Model file for the job. Use its own axes, mm. A direction names the side the tool comes from. Give positions to 0.01 mm unless a question says otherwise; leave off trailing zeros. Loops run counter-clockwise (first coordinate to the right, second up) from the corner with the lowest first, then second, coordinate; pieces in that order, holes last. Notation, with made-up numbers: (10, 72.25) - (43, 72.25) arc R16 ccw to (43, 77.25) - close; hole circle Ø3 at (-3.5, -10). An arc over 180 degrees is marked (long way). Use a Markdown table: item, result.
from build123d import *

# Parameters (mm, degrees)
F0_R     = 40
F0_R_2   = 11
F1_DEPTH = 9
F2_R     = 1
F3_SIZE  = 1
F9_DEPTH = 2.5


with BuildPart() as f1:
    # F0 (on Top) → F1 (new body)
    with BuildSketch(Plane.XY):
        Circle(F0_R)
        Circle(F0_R_2, mode=Mode.SUBTRACT)
    extrude(amount=F1_DEPTH)

    # F2
    f2_edges = [f1.edges().sort_by_distance(p)[0] for p in [
        (-11, 0, 9),
    ]]
    fillet(f2_edges, radius=F2_R)

    # F3
    f3_edges = [f1.edges().sort_by_distance(p)[0] for p in [
        (-11, 0, 0),
    ]]
    chamfer(f3_edges, length=F3_SIZE)

    # F8 (on face) → F9 (join, symmetric)
    with BuildSketch(Plane.XY.offset(4.5)):
        with BuildLine():
            Line((-12, 1.5), (-12, -1.5))
            Line((-12, -1.5), (-10, -1.5))
            ThreePointArc((-10, -1.5), (-9.292893, -1.207107), (-9, -0.5))
            Line((-9, -0.5), (-9, 0.5))
            ThreePointArc((-9, 0.5), (-9.292893, 1.207107), (-10, 1.5))
            Line((-10, 1.5), (-12, 1.5))
        make_face()
        with BuildLine():
            Line((4.700962, -11.142305), (7.299038, -9.642305))
            Line((7.299038, -9.642305), (6.299038, -7.910254))
            ThreePointArc((6.299038, -7.910254), (5.691832, -7.444328), (4.933013, -7.544229))
            Line((4.933013, -7.544229), (4.066987, -8.044229))
            ThreePointArc((4.066987, -8.044229), (3.601061, -8.651435), (3.700962, -9.410254))
            Line((3.700962, -9.410254), (4.700962, -11.142305))
        make_face()
        with BuildLine():
            Line((7.299038, 9.642305), (4.700962, 11.142305))
            Line((4.700962, 11.142305), (3.700962, 9.410254))
            ThreePointArc((3.700962, 9.410254), (3.601061, 8.651435), (4.066987, 8.044229))
            Line((4.066987, 8.044229), (4.933013, 7.544229))
            ThreePointArc((4.933013, 7.544229), (5.691832, 7.444328), (6.299038, 7.910254))
            Line((6.299038, 7.910254), (7.299038, 9.642305))
        make_face()
    extrude(amount=F9_DEPTH, both=True)


solid = f1.part
(1) Slice it at C-C, the plane y = 28. Write the cut outline in (x, z), plus the area to 3 significant figures.
Computed:
| item | result |
|---|---|
| outline | (-28.57, 0) - (28.57, 0) - (28.57, 9) - (-28.57, 9) - close |
| area | 514 mm² |
(2) Pin check, flat tips, straight feed: P1, Ø0.7, axis at x = -10.5, z = 5.5, coming from the +Y side; P2, Ø0.6, axis at x = -10, y = 0, coming from the +Z side; P3, Ø1.4, axis at x = 5, y = 8.5, coming from the -Z side. Stop position of each tip, or through.
Computed:
| item | result |
|---|---|
| P1 | y = 38.69 |
| P2 | z = 7 |
| P3 | z = 2 |
(3) Slice it at D-D, the plane x = -23.5. Write the cut outline in (y, z), plus the area to 3 significant figures.
Computed:
| item | result |
|---|---|
| outline | (-32.37, 0) - (32.37, 0) - (32.37, 9) - (-32.37, 9) - close |
| area | 583 mm² |
(4) Slice it at B-B, the plane x = 0. Write the cut outline in (y, z), plus the area to 3 significant figures.
Computed:
| item | result |
|---|---|
| outline | (-40, 0) - (-12, 0) - (-11, 1) - (-11, 8) arc R1 ccw to (-12, 9) - (-40, 9) - close; (11, 1) - (12, 0) - (40, 0) - (40, 9) - (12, 9) arc R1 ccw to (11, 8) - close |
| area | 521 mm² |
(5) 3-axis set-ups, long thin cutter, end or side, ignore diameter. For faces 4 (the flat face through (8.3, 9.4, 9)), 5 (the flat face through (5, -9, 7)), 6 (the flat face through (-10, 0, 2)): which of +Z, -Z, +X, -X, +Y, -Y reach the whole face in a straight line?
Computed:
| item | result |
|---|---|
| face 4 | +Z, +X, -X, +Y, -Y |
| face 5 | +Z |
| face 6 | -Z |
(6) Slice it at A-A, the plane z = 5.75. Write the cut outline in (x, y), plus the area to 3 significant figures.
Computed:
| item | result |
|---|---|
| outline | circle Ø80 at (0, 0); hole (-10.9, -1.5) arc R11 ccw to (4.15, -10.19) - (3.7, -9.41) arc R1 cw to (4.07, -8.04) - (4.93, -7.54) arc R1 cw to (6.3, -7.91) - (6.75, -8.69) arc R11 ccw to (6.75, 8.69) - (6.3, 7.91) arc R1 cw to (4.93, 7.54) - (4.07, 8.04) arc R1 cw to (3.7, 9.41) - (4.15, 10.19) arc R11 ccw to (-10.9, 1.5) - (-10, 1.5) arc R1 cw to (-9, 0.5) - (-9, -0.5) arc R1 cw to (-10, -1.5) - close |
| area | 4,660 mm² |
(7) Drill centre lines: probe 1 along Y at (x, z) = (0, 5); probe 2 along Y at (x, z) = (4, 5.75); probe 3 along X at (y, z) = (6, 1.5). Where is each one in solid material? Low to high. Write a range as [from, to].
Computed:
| item | result |
|---|---|
| probe 1 | [-40, -11], [11, 40] |
| probe 2 | [-39.8, -10.25], [-9.93, -8.09], [8.09, 9.93], [10.25, 39.8] |
| probe 3 | [-39.55, -9.22], [9.22, 39.55] |
(8) Mould opens along Y. For faces 1 (the cylindrical face through (-8.67, -39.05, 4.44)), 2 (the flat face through (8.3, 9.4, 0)), 3 (the flat face through (5, -9, 2)) say: pulls with the +Y half, pulls with the -Y half, needs draft (parallel to the pull), parting line crosses it, or undercut.
Computed:
| item | result |
|---|---|
| face 1 | parting line crosses it |
| face 2 | needs draft |
| face 3 | undercut |
